Part model, mm, in its own coordinate system. A direction names the side the tool comes from. Give positions to 0.01 mm unless a question says otherwise; leave off trailing zeros. Order: outer loops, then holes, each group sorted by start corner. A loop starts at its lowest first (then second) coordinate and runs counter-clockwise, first axis right, second up.
1. Drop flat-ended pins along their axis: pin 1 Ø1.5 at (y, z) = (-21, 1) entering from -X; pin 2 Ø1.5 at (x, z) = (21.5, 2) entering from -Y; pin 3 Ø0.9 at (x, z) = (-21.5, 1) entering from +Y. Give the stop position or say it passes through.
2. Mould opens along X. For faces 1 (the flat face through (-11.8, -22, 1)), 2 (the flat face through (23, 16, 1)), 3 (the flat face through (-22, 4.1, 1)) say: +X half, -X half, draft (parallel to the pull), parting line (faces both ways), or undercut.
3. Probe line 1 (Y direction, x = -9, z = 2.45). List the from-to ranges inside material, lowest first.
4. Which spindle directions (+Z, -Z, +X, -X, +Y, -Y) get a long thin tool onto all of the face, cutting with end or side? Do faces 4 (the flat face through (-20, 21, 1)), 5 (the flat face through (-20, 8, 1)), 6 (the flat face through (21, 20, 1)). Say none if no direction does.
5. Slice it at A-A on y = 5. List the corners of the cut face in (x, z).
from build123d import *

# Parameters (mm, degrees)
CROQUIS1_W              = 3
CROQUIS1_H              = 8.2
CROQUIS1_W_2            = 8.2
CROQUIS1_H_2            = 3.00257915
CROQUIS1_W_3            = 40
CROQUIS1_H_3            = 40
SALIENTE_EXTRUIR1_DEPTH = 3


with BuildPart() as part:
    # Croquis1 → Saliente-Extruir1 (new body)
    with BuildSketch(Plane.XY):
        with Locations((-21.5, 15.9)):
            Rectangle(CROQUIS1_W, CROQUIS1_H)
        with Locations((-15.9, 21.501289575)):
            Rectangle(CROQUIS1_W_2, CROQUIS1_H_2)
        with Locations((0, 21.501289575)):
            Rectangle(CROQUIS1_W_2, CROQUIS1_H_2)
        with Locations((15.9, 21.501289575)):
            Rectangle(CROQUIS1_W_2, CROQUIS1_H_2)
        Rectangle(CROQUIS1_W_3, CROQUIS1_H_3)
        with Locations((21.5, 0)):
            Rectangle(CROQUIS1_W, CROQUIS1_H)
        with Locations((-21.5, 0)):
            Rectangle(CROQUIS1_W, CROQUIS1_H)
        with Locations((-21.5, -15.9)):
            Rectangle(CROQUIS1_W, CROQUIS1_H)
        with Locations((-15.9, -21.501289575)):
            Rectangle(CROQUIS1_W_2, CROQUIS1_H_2)
        with Locations((0, -21.501289575)):
            Rectangle(CROQUIS1_W_2, CROQUIS1_H_2)
        with Locations((15.9, -21.501289575)):
            Rectangle(CROQUIS1_W_2, CROQUIS1_H_2)
        with Locations((21.5, -15.9)):
            Rectangle(CROQUIS1_W, CROQUIS1_H)
        with Locations((21.5, 15.9)):
            Rectangle(CROQUIS1_W, CROQUIS1_H)
    extrude(amount=SALIENTE_EXTRUIR1_DEPTH)


solid = part.part
Data:
1. pin 1: stops at x = -20
1. pin 2: stops at y = -20
1. pin 3: stops at y = 20
2. face 1: undercut
2. face 2: +X half
2. face 3: draft
3. line 1: y = -20 to 20
4. face 4: +Z, -Z, -X, +Y
4. face 5: +Z, -Z, -X
4. face 6: +Z, -Z, +X, +Y
5. outline: (-20, 0) - (20, 0) - (20, 3) - (-20, 3) - close
